Could you check a few things on this drawing? It's one solid part, dimensions in mm from its lowest x, y, z. A direction names the side the tool comes from. Coordinates: 2 decimals unless noted, no trailing zeros. Loops run counter-clockwise (first coordinate to the right, second up) from the corner with the lowest first, then second, coordinate; pieces in that order, holes last. Notation, with made-up numbers: M 88.25,68.5 L 125.25,68.5 A12 cw 125.25,72.5 Z; hole C -20.5,-32 d5. An arc over 180 degrees is marked long. Use one line per item in the form item = value. Start each with the question number.
(1) Imagine slicing it at A-A, the plane y = 10.5. Please give me the cut outline in (x, z), and give its area (3 significant figures).
(2) Thinking about a two-plate mould opening in X: for the marked faces 1, 2, 3 and 4, which applies, +X half, -X half, draft (parallel to the pull), parting line (faces both ways), or undercut?
(3) Imagine slicing it at B-B, the plane z = 3.75. Please give me the cut outline in (x, y), and give its area (3 significant figures).
(4) Will these pins go through, and if not, where does the flat tip stop? P1, Ø7.5, axis at x = 2, y = 9.5, coming from the +Z side; P2, Ø2.5, axis at x = 49.5, y = 23.5, coming from the +Z side; P3, Ø8, axis at x = 39, y = 3, coming from the +Z side (1 decimal).
(5) Imagine slicing it at D-D, the plane y = 14.75. Please give me the cut outline in (x, z).
(6) On a 3-axis mill with a long thin cutter (end or side, diameter ignored), from which of +Z, -Z, +X, -X, +Y, -Y can I reach the whole of each face in a straight line? I mean the marked faces 5, 6, 7, 8 and 9. Say none if no direction works.
(7) Imagine slicing it at C-C, the plane x = 39. Please give me the cut outline in (y, z).
(8) Please list where these lines run through material, in increasing order: L1, parallel to X at y = 1.5, z = 5.25; L2, parallel to Z at x = 4, y = 11.75; L3, parallel to Z at x = 43.5, y = 18.5.
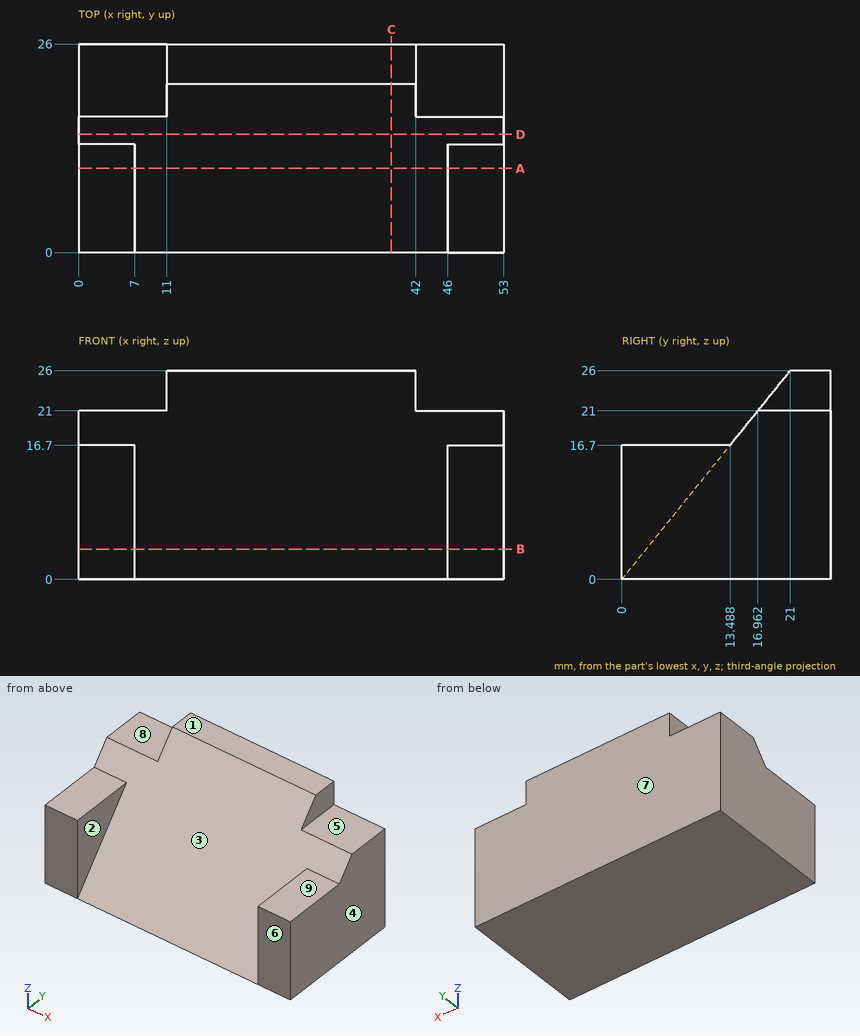
Answer:
q1.outline = M 0,0 L 53,0 L 53,16.7 L 46,16.7 L 46,13 L 7,13 L 7,16.7 L 0,16.7 Z
q1.area = 741 mm²
q2.face_1 = draft
q2.face_2 = undercut
q2.face_3 = undercut
q2.face_4 = +X half
q3.outline = M 0,0 L 7,0 L 7,3.03 L 46,3.03 L 46,0 L 53,0 L 53,26 L 0,26 Z
q3.area = 1,260 mm²
q4.P1 = 16.7
q4.P2 = 21
q4.P3 = 8.7
q5.outline = M 0,0 L 53,0 L 53,18.26 L 0,18.26 Z
q6.face_5 = +Z, +X, +Y, -Y
q6.face_6 = +Z, -Z, +X, -X, -Y
q6.face_7 = +Z, -Z, +X, -X, +Y
q6.face_8 = +Z, -X, +Y, -Y
q6.face_9 = +Z, +X, -X, -Y
q7.outline = M 0,0 L 26,0 L 26,26 L 21,26 Z
q8.L1 = 0 to 7, 46 to 53
q8.L2 = 0 to 16.7
q8.L3 = 0 to 21
